Source: CAD feature listing. Evaluate the final solid. Frame: model axes, mm. A direction names the side the tool comes from. Coordinates: 2 decimals unless noted, no trailing zeros. Order: outer loops, then holes, each group sorted by start corner. A loop starts at its lowest first (then second) coordinate and runs counter-clockwise, first axis right, second up.
Item 1: Section D-D on x = -5.25. Return the cut outline in (y, z), then the cut area to 3 significant figures.
Item 2: Section B-B on x = -2.75. Return the cut outline in (y, z).
Item 3: Contact query for flat-ended pins moving along their axis: P1, Ø1, axis at x = 2, z = 1.5, coming from the +Y side; P2, Ø1.2, axis at x = -3, z = 1.5, coming from the -Y side; P3, Ø1.5, axis at x = 0, z = 2, coming from the +Y side. Output: stop coordinate, or through.
Item 4: Mould query, pull axis Y, two halves, no side actions, for faces 1 (the flat face through (-3, -0.25, 2)), 2 (the flat face through (0, -6.5, 2)), 3 (the flat face through (-3.5, 7, 2)). Classes: released by +Y, released by -Y, zero draft, split by the parting line, or undercut.
Item 5: Reachability of faces 4 (the flat face through (-6, 8.5, 1)), 5 (the flat face through (-3, 5.5, 2)), 6 (the flat face through (4, -2, 2)) from +Z, -Z, +X, -X, +Y, -Y: full face, straight path, thin tool, end or side. Return the list, or none.
Item 6: Section C-C on z = 0.4. Return the cut outline in (x, y), then the cut area to 3 significant figures.
Item 7: Section A-A on y = 3.25. Return the cut outline in (x, z), then the cut area to 3 significant figures.
Item 8: Ray query, line 1 (X direction, y = 4.5, z = 0.8); line 2 (X direction, y = 7, z = 2.1); line 3 (Y direction, x = -2, z = 2.85). Return the intervals inside material, ascending.
from build123d import *

# Parameters (mm, degrees)
SALIENTE_EXTRUIR1_DEPTH = 3
CORTAR_EXTRUIR1_DEPTH   = 10
CROQUIS3_W              = 2
CROQUIS3_H              = 3
CORTAR_EXTRUIR2_DEPTH   = 10
SALIENTE_EXTRUIR2_START = -3
SALIENTE_EXTRUIR2_DEPTH = 3


with BuildPart() as part:
    # Croquis1 → Saliente-Extruir1 (new body)
    with BuildSketch(Plane.XY):
        with BuildLine():
            Line((-7.5, -0.5), (-7.5, 8.5))
            Line((-7.5, 8.5), (7.5, 8.5))
            Line((7.5, 8.5), (7.5, -0.5))
            Line((7.5, -0.5), (5, -3.5))
            Line((5, -3.5), (3, -4.462410552))
            ThreePointArc((3, -4.462410552), (0, -7.462410552), (-3, -4.462410552))
            Line((-3, -4.462410552), (-5, -3.5))
            Line((-5, -3.5), (-7.5, -0.5))
        make_face()
    extrude(amount=SALIENTE_EXTRUIR1_DEPTH)

    # Croquis2 → Cortar-Extruir1 (cut)
    with BuildSketch(Plane.XY.offset(3)):
        Polygon((1.5, 8.5), (-1.5, 8.5), (-1.5, -0.25), (-4, -0.25), (-4, -3.25), (-1.5, -3.25), (-1.5, -6.5), (1.5, -6.5), (1.5, -3.25), (4, -3.25), (4, -0.25), (1.5, -0.25), align=None)
    extrude(amount=-CORTAR_EXTRUIR1_DEPTH, mode=Mode.SUBTRACT)

    # Croquis3 → Cortar-Extruir2 (cut)
    with BuildSketch(Plane.XY.offset(3)):
        with Locations((-2.5, 7)):
            Rectangle(CROQUIS3_W, CROQUIS3_H)
        with Locations((2.5, 7)):
            Rectangle(CROQUIS3_W, CROQUIS3_H)
    extrude(amount=-CORTAR_EXTRUIR2_DEPTH, mode=Mode.SUBTRACT)

    # Croquis5 → Saliente-Extruir2 (add)
    with BuildSketch(Plane.XY.offset(3).offset(SALIENTE_EXTRUIR2_START)):
        with BuildLine():
            ThreePointArc((-7.440502446, -0.571397065), (-7.422411846, -0.771604582), (-7.39893509, -0.971252175))
            Line((-7.39893509, -0.971252175), (-7.146532031, -2.148173916))
            ThreePointArc((-7.146532031, -2.148173916), (-4.452921263, -5.988243772), (0, -7.462410552))
            ThreePointArc((0, -7.462410552), (-2.121320344, -6.583730896), (-3, -4.462410552))
            Line((-3, -4.462410552), (-5, -3.5))
            Line((-5, -3.5), (-7.440502446, -0.571397065))
        make_face()
        with BuildLine():
            ThreePointArc((3, -4.462410552), (2.121320344, -6.583730896), (0, -7.462410552))
            ThreePointArc((0, -7.462410552), (5.070679035, -5.475014646), (7.440502446, -0.571397065))
            Line((7.440502446, -0.571397065), (5, -3.5))
            Line((5, -3.5), (3, -4.462410552))
        make_face()
    extrude(amount=SALIENTE_EXTRUIR2_DEPTH)


solid = part.part
Answer list:
1. outline: (-5.3, 0) - (8.5, 0) - (8.5, 3) - (-5.3, 3) - close
1. area: 41.4 mm2
2. outline: (-6.94, 0) - (-3.25, 0) - (-3.25, 3) - (-6.94, 3) - close; (-0.25, 0) - (5.5, 0) - (5.5, 3) - (-0.25, 3) - close
3. P1: stops at y = 5.5
3. P2: stops at y = -7.07
3. P3: stops at y = -6.5
4. face 1: undercut
4. face 2: released by +Y
4. face 3: zero draft
5. face 4: +Z, -Z, +X, -X, +Y
5. face 5: +Z, -Z, +Y
5. face 6: +Z, -Z
6. outline: (-7.5, -0.5) - (-7.44, -0.57) arc R7.46 ccw to (-7.4, -0.97) - (-7.15, -2.15) arc R7.46 ccw to (7.44, -0.57) - (7.5, -0.5) - (7.5, 8.5) - (3.5, 8.5) - (3.5, 5.5) - (1.5, 5.5) - (1.5, -0.25) - (4, -0.25) - (4, -3.25) - (1.5, -3.25) - (1.5, -6.5) - (-1.5, -6.5) - (-1.5, -3.25) - (-4, -3.25) - (-4, -0.25) - (-1.5, -0.25) - (-1.5, 5.5) - (-3.5, 5.5) - (-3.5, 8.5) - (-7.5, 8.5) - close
6. area: 143 mm2
7. outline: (-7.5, 0) - (-1.5, 0) - (-1.5, 3) - (-7.5, 3) - close; (1.5, 0) - (7.5, 0) - (7.5, 3) - (1.5, 3) - close
7. area: 36.0 mm2
8. line 1: x = -7.5 to -1.5, 1.5 to 7.5
8. line 2: x = -7.5 to -3.5, 3.5 to 7.5
8. line 3: y = -7.19 to -3.25, -0.25 to 5.5
